Can you work these out from the model? Positions are in its coordinate system, mm. A direction names the side the tool comes from. Coordinates: 2 decimals unless noted, no trailing zeros. Loops run counter-clockwise (first coordinate to the right, second up) from the corner with the lowest first, then second, coordinate; pieces in that order, holes last.
```python
from build123d import *

# Parameters (mm, degrees)
PAD_DEPTH = 9


with BuildPart() as part:
    # Sketch → Pad (new body)
    with BuildSketch(Plane.XY):
        with BuildLine():
            Line((-1.75, 13.638182), (-4, 16.838182))
            Line((-1.4, 16.838182), (-4, 16.838182))
            ThreePointArc((-1.4, 16.838182), (0, 15.438182), (1.4, 16.838182))
            Line((1.4, 16.838182), (4, 16.838182))
            Line((4, 16.838182), (1.75, 13.638182))
            ThreePointArc((-1.75, 13.638182), (0, -13.75), (1.75, 13.638182))
        make_face()
        Polygon((-6.43, 10.068182), (6.43, 10.068182), (11.93, 0.541902), (5.5, -10.595184), (-5.5, -10.595184), (-11.93, 0.541902), align=None, mode=Mode.SUBTRACT)
    extrude(amount=PAD_DEPTH)


solid = part.part
```
(1) I'm going to push flat-ended pins straight in: pin 1 (1.5 mm diameter, centred on y = 2.5, z = 2, fed in from -X); pin 2 (3 mm diameter, centred on x = -2.5, z = 4, fed in from -Y); pin 3 (2 mm diameter, centred on x = 2, y = -9, fed in from -Z); pin 4 (5 mm diameter, centred on y = 12.5, z = 7, fed in from +X). Where does each tip first touch, or does it pass through?
Check values:
pin 1: stops at x = -13.64
pin 2: stops at y = -13.71
pin 3: passes through
pin 4: stops at x = 9.44
(2) If we mould it in two halves opening along Y, with no side actions, what happens to faces 1 (the flat face through (2.89, 15.26, 4.44)), 2 (the flat face through (3, 16.838, 4)), 3 (the flat face through (0, 11, 9))? For each: released by +Y, released by -Y, zero draft, split by the parting line, or undercut.
Check values:
face 1: undercut
face 2: released by +Y
face 3: zero draft
(3) Which directions (+Z, -Z, +X, -X, +Y, -Y) give clear straight access to the entire face, cutting with the end or side of a thin tool? Please do faces 4 (the flat face through (8.76, -4.95, 4.44)), 5 (the flat face through (-3, 16.838, 4)), 6 (the flat face through (-2.86, 15.22, 4.44)).
Check values:
face 4: +Z, -Z
face 5: +Z, -Z, +X, -X, +Y
face 6: +Z, -Z, -X
(4) I want a section at D-D on x = -3. Write out the boundary of the cut face in (y, z), then the cut area to 3 significant figures.
Check values:
outline: (-13.42, 0) - (-10.6, 0) - (-10.6, 9) - (-13.42, 9) - close; (10.07, 0) - (13.42, 0) - (13.42, 9) - (10.07, 9) - close; (15.42, 0) - (16.84, 0) - (16.84, 9) - (15.42, 9) - close
area: 68.4 mm2
(5) I want a section at A-A on x = 0. Write out the boundary of the cut face in (y, z).
Check values:
outline: (-13.75, 0) - (-10.6, 0) - (-10.6, 9) - (-13.75, 9) - close; (10.07, 0) - (15.44, 0) - (15.44, 9) - (10.07, 9) - close
(6) If I drill on probe 1 along Y at (x, z) = (0, 7.5); probe 2 along Y at (x, z) = (-7.5, 8); probe 3 along X at (y, z) = (-8, 8.5), over which ranges is the centre line in solid material (lowest first)?
Check values:
probe 1: y = -13.75 to -10.6, 10.07 to 15.44
probe 2: y = -11.52 to -7.13, 8.21 to 11.52
probe 3: x = -11.18 to -7, 7 to 11.18
(7) I want a section at B-B on y = 6.5. Write out the boundary of the cut face in (x, z), then the cut area to 3 significant figures.
Check values:
outline: (-12.12, 0) - (-8.49, 0) - (-8.49, 9) - (-12.12, 9) - close; (8.49, 0) - (12.12, 0) - (12.12, 9) - (8.49, 9) - close
area: 65.3 mm2
(8) I want a section at C-C on z = 1.25. Write out the boundary of the cut face in (x, y), then the cut area to 3 significant figures.
Check values:
outline: (-4, 16.84) - (-1.75, 13.64) arc R13.75 ccw (long way) to (1.75, 13.64) - (4, 16.84) - (1.4, 16.84) arc R1.4 cw to (-1.4, 16.84) - close; hole (-11.93, 0.54) - (-5.5, -10.6) - (5.5, -10.6) - (11.93, 0.54) - (6.43, 10.07) - (-6.43, 10.07) - close
area: 240 mm2
